For this review, take the finished solid that the model builds, in its own axes (mm). A direction names the side the tool comes from. Round coordinates to 2 decimals unless told otherwise and drop trailing zeros. Write each loop counter-clockwise with the first axis right and the second up, starting at its lowest first coordinate (ties: lowest second). Pieces come first, ordered by that corner, then holes. Notation, with made-up numbers: M 85,-37 L 144,-37 A5 cw 144,-32 Z; hole C 82.5,-24.5 d1. An arc over 180 degrees is marked long. Answer in a Markdown table with one row per item.
```python
from build123d import *

# Parameters (mm, degrees)
F0_W     = 3
F0_H     = 16
F1_DEPTH = 10
F2_W     = 8
F2_H     = 3
F3_DEPTH = 25
F4_W     = 30
F4_H     = 16
F5_DEPTH = 5
F7_DEPTH = 50
F6_W     = 10
F6_H     = 29
F8_DEPTH = 5
F9_R     = 2
F10_R    = 3
F11_R    = 1


with BuildPart() as f1:
    # F0 (on Top) → F1 (new body)
    with BuildSketch(Plane.XY):
        with Locations((-5, 8)):
            Rectangle(F0_W, F0_H)
    extrude(amount=F1_DEPTH)


with BuildPart() as f1b:
    # F0 (on Top) → F1, piece 2 (new body)
    with BuildSketch(Plane.XY):
        with Locations((5, 8)):
            Rectangle(F0_W, F0_H)
    extrude(amount=F1_DEPTH)


with BuildPart() as f3_tool:
    # F2 (on face) → F3 (new body)
    with BuildSketch(Plane(origin=(-6.5, 0, 0), x_dir=(0, -1, 0), z_dir=(-1, 0, 0))):
        with Locations((-4, 1.5)):
            Rectangle(F2_W, F2_H)
    extrude(amount=-F3_DEPTH)


with BuildPart() as f1_1:
    add(f1.part)

    # F3: cut by f3_tool
    add(f3_tool.part, mode=Mode.SUBTRACT)



with BuildPart() as f1b_1:
    add(f1b.part)

    # F3: cut by f3_tool
    add(f3_tool.part, mode=Mode.SUBTRACT)


with BuildPart() as f1_2:
    add(f1_1.part)

    add(f1b_1.part)  # F5 merges F1b
    # F4 (on Top) → F5 (join)
    with BuildSketch(Plane.XY):
        with Locations((-3.5, 8)):
            Rectangle(F4_W, F4_H)
    extrude(amount=-F5_DEPTH)

    # F6 (on Front) → F7 (join)
    with BuildSketch(Plane.XZ):
        Polygon((-113.5, -18), (-123.5, -18), (-123.5, 11), (-113.5, 11), (-31.5, 11), (-21.5, 11), (-21.5, -18), (-31.5, -18), (-38.5, -18), (-38.5, -21), (-18.5, -21), (-18.5, 14), (-126.5, 14), (-126.5, -21), (-106.5, -21), (-106.5, -18), align=None)
    extrude(amount=-F7_DEPTH)

    # F6 (on Front) → F8 (join)
    with BuildSketch(Plane.XZ):
        with Locations((-26.5, -3.5)):
            Rectangle(F6_W, F6_H)
        with Locations((-118.5, -3.5)):
            Rectangle(F6_W, F6_H)
    extrude(amount=-F8_DEPTH)

    # F9
    f9_edges = [f1_2.edges().sort_by_distance(p)[0] for p in [
        (-5, 16, 10),
        (5, 16, 10),
        (-5, 0, 10),
        (5, 0, 10),
        (-5, 0, 3),
        (5, 0, 3),
    ]]
    fillet(f9_edges, radius=F9_R)

    # F10
    f10_edges = [f1_2.edges().sort_by_distance(p)[0] for p in [
        (-21.5, 27.5, 11),
        (-123.5, 27.5, 11),
        (-126.5, 25, 14),
        (-18.5, 25, 14),
        (-18.5, 25, -21),
        (-21.5, 27.5, -18),
        (-123.5, 27.5, -18),
        (-126.5, 25, -21),
        (-123.5, 5, -3.5),
        (-118.5, 5, -18),
        (-26.5, 5, -18),
        (-21.5, 5, -3.5),
        (-26.5, 5, 11),
        (-118.5, 5, 11),
        (-38.5, 0, -19.5),
        (-106.5, 0, -19.5),
        (-38.5, 50, -19.5),
        (-106.5, 50, -19.5),
    ]]
    fillet(f10_edges, radius=F10_R)

    # F11
    f11_edges = [f1_2.edges().sort_by_distance(p)[0] for p in [
        (-18.5, 16, -2.5),
        (-3.5, 16, -5),
        (-12.5, 16, 0),
        (0, 16, 0),
        (9, 16, 0),
        (-18.5, 8, -5),
        (-18.5, 8, 0),
    ]]
    fillet(f11_edges, radius=F11_R)


solid = f1_2.part
```
Q1. Insertion check: P1, Ø0.9, axis at x = 5, y = 6, coming from the +Z side; P2, Ø3.5, axis at y = 33, z = -20, coming from the -X side; P3, Ø3.5, axis at x = -27, z = -5.5, coming from the +Y side; P4, Ø8, axis at x = -37.5, z = -4.5, coming from the +Y side. Each pin has a flat end and moves straight along its axis. Give the tip position at first contact, or say it passes through.
Found:
| item | result |
|---|---|
| P1 | z = 10 |
| P2 | x = -126.49 |
| P3 | y = 5 |
| P4 | through |
Q2. Take a section at B-B (z = -11). State the section outline as (x, y) points, then the cut area to 3 significant figures.
Found:
| item | result |
|---|---|
| outline | M -126.5,0 L -113.5,0 L -113.5,5 L -120.5,5 A3 cw -123.5,8 L -123.5,50 L -126.5,50 Z; M -31.5,0 L -18.5,0 L -18.5,50 L -21.5,50 L -21.5,8 A3 cw -24.5,5 L -31.5,5 Z |
| area | 404 mm² |
Q3. For probe 1 along X at (y, z) = (9.5, 7.5); probe 2 along X at (y, z) = (25.5, -11); probe 3 along X at (y, z) = (4.5, -16), list the stretches that pass through material, from the lowest coordinate up.
Found:
| item | result |
|---|---|
| probe 1 | -126.5 to -123.5, -21.5 to -18.5, -6.5 to -3.5, 3.5 to 6.5 |
| probe 2 | -126.5 to -123.5, -21.5 to -18.5 |
| probe 3 | -126.5 to -113.5, -31.5 to -18.5 |
Q4. Take a section at C-C (y = 45.5). State the section outline as (x, z) points, then the cut area to 3 significant figures.
Found:
| item | result |
|---|---|
| outline | M -126.5,-18 A3 ccw -123.5,-21 L -106.5,-21 L -106.5,-18 L -120.5,-18 A3 cw -123.5,-15 L -123.5,8 A3 cw -120.5,11 L -24.5,11 A3 cw -21.5,8 L -21.5,-15 A3 cw -24.5,-18 L -38.5,-18 L -38.5,-21 L -21.5,-21 A3 ccw -18.5,-18 L -18.5,11 A3 ccw -21.5,14 L -123.5,14 A3 ccw -126.5,11 Z |
| area | 618 mm² |
Q5. Take a section at A-A (x = -30). State the section outline as (y, z) points, then the cut area to 3 significant figures.
Found:
| item | result |
|---|---|
| outline | M 0,-21 L 50,-21 L 50,-18 L 8,-18 A3 cw 5,-15 L 5,8 A3 cw 8,11 L 50,11 L 50,14 L 0,14 Z |
| area | 449 mm² |
Q6. Take a section at D-D (x = -92.5). State the section outline as (y, z) points, then the cut area to 3 significant figures.
Found:
| item | result |
|---|---|
| outline | M 0,11 L 50,11 L 50,14 L 0,14 Z |
| area | 150 mm² |
Q7. Mouldability with a two-part tool opening along X and no side actions: class faces 5 (the face through (11.5, 8, -2)), 6 (the face through (-113, 25, -18)), 7 (the face through (-3, 16, -2)) as +X half, -X half, draft (parallel to the pull), parting line (faces both ways), or undercut.
Found:
| item | result |
|---|---|
| face 5 | +X half |
| face 6 | undercut |
| face 7 | draft |
Q8. Machinability: for faces 1 (the face through (-116.95, 5.9, 10.14)), 2 (the face through (-107.4, 49.14, -19.48)), 3 (the face through (-5, 8, 1)), 4 (the face through (-107.4, 0.86, -19.48)), which of the approach directions +Z, -Z, +X, -X, +Y, -Y give a long, thin tool a straight path to every point of the face, cutting with its end or side? Answer none if there is none.
Found:
| item | result |
|---|---|
| face 1 | +Y |
| face 2 | -Z, +Y |
| face 3 | +X, -Y |
| face 4 | -Z, -Y |
